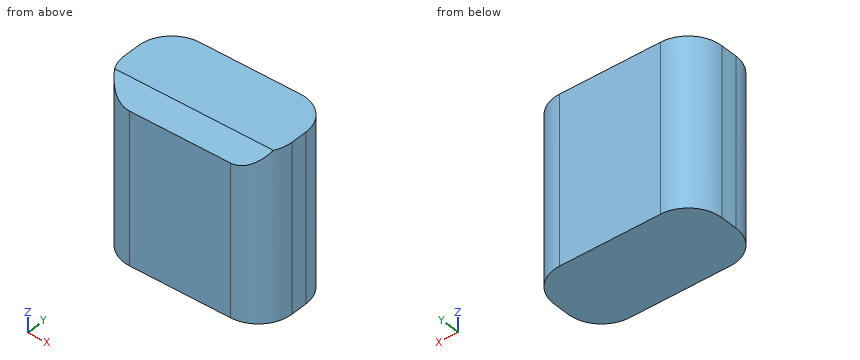
```python
from build123d import *

# Parameters (mm, degrees)
F0_W        = 25.4
F0_H        = 12.7
F1_DEPTH    = 25.4
F2_R        = 5.08
F3_T1_DEPTH = 28.3041495789


# Not quite as in the source:
# - a fillet or chamfer that OpenCascade refuses, or shapes differently, is made with other operations: its cross-section is extruded or revolved along the edge and cut away or added


with BuildPart() as f1:
    # F0 (on Top) → F1 (new body)
    with BuildSketch(Plane.XY):
        with Locations((-7.3743816465, 11.2398102205)):
            Rectangle(F0_W, F0_H)
    extrude(amount=F1_DEPTH)

    # F2
    f2_edges = [f1.edges().sort_by_distance(p)[0] for p in [
        (5.325618, 4.88981, 12.7),
        (5.325618, 17.58981, 12.7),
        (-20.074382, 17.58981, 12.7),
        (-20.074382, 4.88981, 12.7),
    ]]
    fillet(f2_edges, radius=F2_R)

    # F3: chamfer of 2.54 on 1 edges, made by hand

    # F3_s2 → F3_t1 (cut)
    with BuildSketch(Plane.YZ.offset(-21.5264564359)):
        Polygon((7.4298102205, 25.4), (4.8898102205, 22.86), (4.8898102205, 25.4), align=None)
    extrude(amount=F3_T1_DEPTH, mode=Mode.SUBTRACT)


solid = f1.part
```
Here's how the part is built. I have some questions about the finished solid (model axes, mm). Coordinates: 2 decimals unless noted, no trailing zeros. Loops run counter-clockwise (first coordinate to the right, second up) from the corner with the lowest first, then second, coordinate; pieces in that order, holes last. Notation, with made-up numbers: (-26.75, 61.5) -> (8.25, 61.5) arc R16 cw to (8.25, 79.5) -> close; hole circle Ø4 at (84, 89). An arc over 180 degrees is marked (long way). Return JSON: item names as keys, results as strings.
1) Will this pin go through, and if not, where does the flat tip stop? pin 1 (3 mm diameter, centred on y = 7, z = 22.5, fed in from +X).
Results below:
{"pin 1": "x = 5.11"}
2) If we section it at A-A, the plane z = 18.75: Write out the boundary of the cut face in (x, y).
Results below:
{"outline": "(-20.07, 9.97) arc R5.08 ccw to (-14.99, 4.89) -> (0.25, 4.89) arc R5.08 ccw to (5.33, 9.97) -> (5.33, 12.51) arc R5.08 ccw to (0.25, 17.59) -> (-14.99, 17.59) arc R5.08 ccw to (-20.07, 12.51) -> close"}
3) If we section it at D-D, the plane y = 14.5: Write out the boundary of the cut face in (x, z), then the cut area to 3 significant figures.
Results below:
{"outline": "(-19.67, 0) -> (4.92, 0) -> (4.92, 25.4) -> (-19.67, 25.4) -> close", "area": "625 mm²"}
4) I need wall thicknesses on line 1 (X direction, y = 8.25, z = 18.5); line 2 (Z direction, x = -16.25, y = 6.5); line 3 (X direction, y = 12.75, z = 8.5). Which ranges of each line are inside material? Lowest first, please. Write a range as from..to.
Results below:
{"line 1": "-19.77..5.03", "line 2": "0..24.47", "line 3": "-20.07..5.32"}
5) If we section it at C-C, the plane y = 7.75: Write out the boundary of the cut face in (x, z).
Results below:
{"outline": "(-19.56, 0) -> (4.81, 0) -> (4.81, 25.4) -> (-19.56, 25.4) -> close"}
6) If we section it at B-B, the plane x = -16.25: Write out the boundary of the cut face in (y, z), then the cut area to 3 significant figures.
Results below:
{"outline": "(5.05, 0) -> (17.43, 0) -> (17.43, 25.4) -> (7.43, 25.4) -> (5.05, 23.02) -> close", "area": "312 mm²"}
